Can you work these out from the model? Positions are in its coordinate system, mm. A direction names the side the tool comes from. Round coordinates to 2 decimals unless told otherwise and drop trailing zeros. Loops run counter-clockwise (first coordinate to the right, second up) from the corner with the lowest first, then second, coordinate; pieces in that order, holes last.
from build123d import *

# Parameters (mm, degrees)
BOSS_EXTRUDE1_DEPTH = 60.325
SKETCH5_W           = 31.75
SKETCH5_H           = 34.925
CUT_EXTRUDE1_DEPTH  = 77.2
BOSS_EXTRUDE2_DEPTH = 15.875
FILLET1_R           = 12.7
SKETCH7_R           = 6.35
CUT_EXTRUDE2_DEPTH  = 18.4625


with BuildPart() as part:
    # Sketch1 → Boss-Extrude1 (new body)
    with BuildSketch(Plane(origin=(0, 0, 0), x_dir=(0, 0, -1), z_dir=(1, 0, 0))):
        with BuildLine():
            Line((-60.325, 52.3875), (-15.875, 52.3875))
            ThreePointArc((-15.875, 52.3875), (-4.649679849, 47.737820151), (0, 36.5125))
            Line((0, 36.5125), (0, 0))
            Line((0, 0), (-76.2, 0))
            Line((-76.2, 0), (-76.2, 36.5125))
            ThreePointArc((-76.2, 36.5125), (-71.550320151, 47.737820151), (-60.325, 52.3875))
        make_face()
        with BuildLine():
            Line((-60.325, 42.8625), (-15.875, 42.8625))
            ThreePointArc((-15.875, 42.8625), (-9.525, 36.5125), (-15.875, 30.1625))
            Line((-15.875, 30.1625), (-60.325, 30.1625))
            ThreePointArc((-60.325, 30.1625), (-66.675, 36.5125), (-60.325, 42.8625))
        make_face(mode=Mode.SUBTRACT)
    extrude(amount=BOSS_EXTRUDE1_DEPTH)

    # Sketch5 → Cut-Extrude1 (cut, through all)
    with BuildSketch(Plane.XY.offset(76.2)):
        with Locations((30.1625, 34.925)):
            Rectangle(SKETCH5_W, SKETCH5_H)
    extrude(amount=-CUT_EXTRUDE1_DEPTH, mode=Mode.SUBTRACT)

    # Sketch6 → Boss-Extrude2 (add)
    with BuildSketch(Plane.XZ):
        with BuildLine():
            Line((0, 15.875), (0, 60.325))
            Line((0, 60.325), (-47.625, 60.325))
            ThreePointArc((-47.625, 60.325), (-31.909551788, 53.815448212), (-25.4, 38.1))
            ThreePointArc((-25.4, 38.1), (-31.909551788, 22.384551788), (-47.625, 15.875))
            Line((-47.625, 15.875), (0, 15.875))
        make_face()
        with BuildLine():
            ThreePointArc((-25.4, 38.1), (-31.909551788, 53.815448212), (-47.625, 60.325))
            Line((-47.625, 60.325), (-47.625, 42.8625))
            ThreePointArc((-47.625, 42.8625), (-44.257403955, 41.467596045), (-42.8625, 38.1))
            ThreePointArc((-42.8625, 38.1), (-44.257403955, 34.732403955), (-47.625, 33.3375))
            Line((-47.625, 33.3375), (-47.625, 15.875))
            ThreePointArc((-47.625, 15.875), (-31.909551788, 22.384551788), (-25.4, 38.1))
        make_face()
        with BuildLine():
            Line((-47.625, 42.8625), (-47.625, 60.325))
            ThreePointArc((-47.625, 60.325), (-69.85, 38.1), (-47.625, 15.875))
            Line((-47.625, 15.875), (-47.625, 33.3375))
            ThreePointArc((-47.625, 33.3375), (-52.3875, 38.1), (-47.625, 42.8625))
        make_face()
    extrude(amount=-BOSS_EXTRUDE2_DEPTH)

    # Fillet1
    fillet1_edges = [part.edges().sort_by_distance(p)[0] for p in [
        (0, 7.9375, 15.875),
        (0, 7.9375, 60.325),
    ]]
    fillet(fillet1_edges, radius=FILLET1_R)

    # Sketch7 → Cut-Extrude2 (cut, through all)
    with BuildSketch(Plane(origin=(0, 17.4625, 0), x_dir=(1, 0, 0), z_dir=(0, 1, 0))):
        with Locations((30.1625, -15.875)):
            Circle(SKETCH7_R)
        with Locations((30.1625, -60.325)):
            Circle(SKETCH7_R)
    extrude(amount=-CUT_EXTRUDE2_DEPTH, mode=Mode.SUBTRACT)


solid = part.part
(1) If we section it at B-B, the plane z = 26: List the corners of the cut face in (x, y) for me (1 decimal).
Worked answers:
outline: (-66.3, 0) - (60.3, 0) - (60.3, 30.2) - (46, 30.2) - (46, 17.5) - (14.3, 17.5) - (14.3, 30.2) - (0, 30.2) - (0, 15.9) - (-66.3, 15.9) - close; (0, 42.9) - (14.3, 42.9) - (14.3, 52.4) - (0, 52.4) - close; (46, 42.9) - (60.3, 42.9) - (60.3, 52.4) - (46, 52.4) - close
(2) For faces 4 (the flat face through (7, 42.862, 38)), 5 (the flat face through (30, 14, 0)), 6 (the flat face through (14.288, 27, 39)), 7 (the flat face through (-35, 15.875, 39)), which set-ups out of +Z, -Z, +X, -X, +Y, -Y let a thin tool reach every point of the face, with its end or its side?
Worked answers:
face 4: +X, -X
face 5: -Z, +X, -X, +Y, -Y
face 6: +Z, -Z, +Y
face 7: +Z, -Z, -X, +Y
(3) If we section it at A-A, the plane y = 5.5: State how many separate pieces and enclosed holes the cut face has, then the cut area to 3 significant figures.
Worked answers:
separate pieces: 1
enclosed holes: 3
area: 7,230 mm2
(4) If I drill on line 1 (X direction, y = 30, z = 48) (1 decimal); line 2 (Y direction, x = 3.5, z = 32.5); line 3 (Z direction, x = 49, y = 36), over which ranges is the centre line in solid material (lowest first)?
Worked answers:
line 1: x = 0 to 14.3, 46 to 60.3
line 2: y = 0 to 30.16, 42.86 to 52.39
line 3: z = 0 to 9.55, 66.65 to 76.2
(5) Will these pins go through, and if not, where does the flat tip stop? P1, Ø9.5, axis at x = 27.5, z = 21, coming from the +Y side; P2, Ø8, axis at x = -51, y = 16, coming from the +Z side (3 decimals); P3, Ø1, axis at x = -5.5, z = 26.5, coming from the -Y side; P4, Ø12.5, axis at x = -28.5, y = 8, coming from the -Z side (3 decimals).
Worked answers:
P1: stops at y = 17.46
P2: stops at z = 60.325
P3: stops at y = 0
P4: stops at z = 15.875
(6) If we mould it in two halves opening along Z, with no side actions, what happens to faces 1 (the cylindrical face through (-3.622, 8.049, 12.056)), 2 (the flat face through (53, 30.162, 38)), 3 (the flat face through (0, 27, 38))? For each: released by +Z, released by -Z, zero draft, split by the parting line, or undercut.
Worked answers:
face 1: released by -Z
face 2: undercut
face 3: zero draft
(7) If we section it at D-D, the plane x = 34: List the corners of the cut face in (y, z) for me, then the cut area to 3 significant figures.
Worked answers:
outline: (0, 0) - (17.46, 0) - (17.46, 10.82) - (0, 10.82) - close; (0, 20.93) - (17.46, 20.93) - (17.46, 55.27) - (0, 55.27) - close; (0, 65.38) - (17.46, 65.38) - (17.46, 76.2) - (0, 76.2) - close
area: 977 mm2
(8) If we section it at C-C, the plane y = 41.5: List the corners of the cut face in (x, z) for me (1 decimal).
Worked answers:
outline: (0, 0.8) - (14.3, 0.8) - (14.3, 11.9) - (0, 11.9) - close; (0, 64.3) - (14.3, 64.3) - (14.3, 75.4) - (0, 75.4) - close; (46, 0.8) - (60.3, 0.8) - (60.3, 11.9) - (46, 11.9) - close; (46, 64.3) - (60.3, 64.3) - (60.3, 75.4) - (46, 75.4) - close
